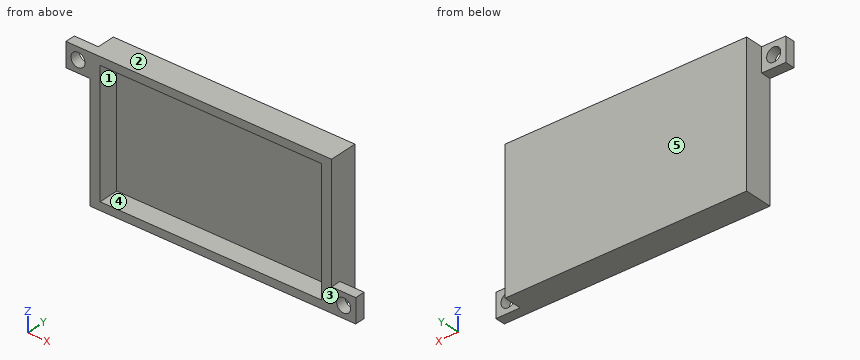
```python
from build123d import *

# Parameters (mm, degrees)
SKETCH1_W           = 60
SKETCH1_H           = 35
BOSS_EXTRUDE1_DEPTH = 7
SKETCH3_W           = 6
SKETCH3_H           = 6
SKETCH3_R           = 1.75
BOSS_EXTRUDE2_DEPTH = 2.5
SKETCH4_W           = 55
SKETCH4_H           = 31
CUT_EXTRUDE1_DEPTH  = 5


with BuildPart() as part:
    # Sketch1 → Boss-Extrude1 (new body)
    with BuildSketch(Plane(origin=(0, 0, 0), x_dir=(1, 0, 0), z_dir=(0, 1, 0))):
        Rectangle(SKETCH1_W, SKETCH1_H)
    extrude(amount=BOSS_EXTRUDE1_DEPTH)

    # Sketch3 → Boss-Extrude2 (add)
    with BuildSketch(Plane(origin=(0, 0, 0), x_dir=(1, 0, 0), z_dir=(0, 1, 0))):
        with Locations((-33, -14.5)):
            Rectangle(SKETCH3_W, SKETCH3_H)
        with Locations(Location((-33, -14.5, 0), (0, 0, 90))):  # turned: the seam where the file's is
            Circle(SKETCH3_R, mode=Mode.SUBTRACT)
        with Locations((33, 14.5)):
            Rectangle(SKETCH3_W, SKETCH3_H)
        with Locations(Location((33, 14.5, 0), (0, 0, 90))):  # turned: the seam where the file's is
            Circle(SKETCH3_R, mode=Mode.SUBTRACT)
    extrude(amount=BOSS_EXTRUDE2_DEPTH)

    # Sketch4 → Cut-Extrude1 (cut)
    with BuildSketch(Plane(origin=(0, 0, 0), x_dir=(-1, 0, 0), z_dir=(0, -1, 0))):
        Rectangle(SKETCH4_W, SKETCH4_H)
    extrude(amount=-CUT_EXTRUDE1_DEPTH, mode=Mode.SUBTRACT)


solid = part.part
```
Could you check a few things on this model? Use its own coordinates, in mm. Face numbers are marked on the shaded views. A direction names the side the tool comes from. Coordinates: 2 decimals unless noted, no trailing zeros. Write each loop counter-clockwise with the first axis right and the second up, starting at its lowest first coordinate (ties: lowest second). Pieces come first, ordered by that corner, then holes. Notation, with made-up numbers: M 85.5,-22 L 99.5,-22 A15 cw 99.5,-16 Z; hole C 58,14.25 d1. An arc over 180 degrees is marked long. Answer as CSV lines item,"result". Start each with the question number.
1) I want a section at C-C, the plane y = 4. Please give me the cut outline in (x, z).
2) I want a section at A-A, the plane x = -33. Please give me the cut outline in (y, z), and give its area (3 significant figures).
3) For P1, Ø2, axis at y = 4.5, z = 4.5, coming from the +X side; P2, Ø0.8, axis at x = 32.5, y = 0.5, coming from the +Z side; P3, Ø9.5, axis at x = 2, z = 4, coming from the -Y side, each with a flat end and sliding along its axis, tell me the tip position at first contact or that it passes through.
4) We'd pull the mould along Z, two halves only. Please class the marked faces 1, 2 and 3: +Z half, -Z half, draft (parallel to the pull), parting line (faces both ways), or undercut.
5) I want a section at B-B, the plane z = 14.5. Please give me the cut outline in (x, y).
6) Please list where these lines run through material, in increasing order: line 1 (X direction, y = 1.5, z = -1); line 2 (X direction, y = 0.7, z = -14.5); line 3 (Z direction, x = -23.5, y = 4.25). Write a range as from..to.
7) For the marked faces 4 and 5, which set-ups out of +Z, -Z, +X, -X, +Y, -Y let a thin tool reach every point of the face, with its end or its side?
Data:
1,outline,"M -30,-17.5 L 30,-17.5 L 30,17.5 L -30,17.5 Z; hole M -27.5,-15.5 L 27.5,-15.5 L 27.5,15.5 L -27.5,15.5 Z"
2,outline,"M 0,11.5 L 2.5,11.5 L 2.5,12.75 L 0,12.75 Z; M 0,16.25 L 2.5,16.25 L 2.5,17.5 L 0,17.5 Z"
2,area,"6.25 mm^2"
3,P1,"stops at x = 30"
3,P2,"stops at z = -11.5"
3,P3,"stops at y = 5"
4,face 1,"undercut"
4,face 2,"+Z half"
4,face 3,"draft"
5,outline,"M -36,0 L -34.75,0 L -34.75,2.5 L -36,2.5 Z; M -31.25,0 L -27.5,0 L -27.5,5 L 27.5,5 L 27.5,0 L 30,0 L 30,7 L -30,7 L -30,2.5 L -31.25,2.5 Z"
6,line 1,"x = -30..-27.5, 27.5..30"
6,line 2,"x = -30..-27.5, 27.5..31.25, 34.75..36"
6,line 3,"z = -17.5..-15.5, 15.5..17.5"
7,face 4,"-Y"
7,face 5,"+Z, -Z, +X, -X, +Y"
